Check sheet for the drawn part. Datum: minimum x, y, z corner. Units: mm. A direction names the side the tool comes from. Give positions to 0.01 mm unless a question says otherwise; leave off trailing zeros. Order: outer loops, then holes, each group sorted by start corner. A loop starts at its lowest first (then second) coordinate and runs counter-clockwise, first axis right, second up.
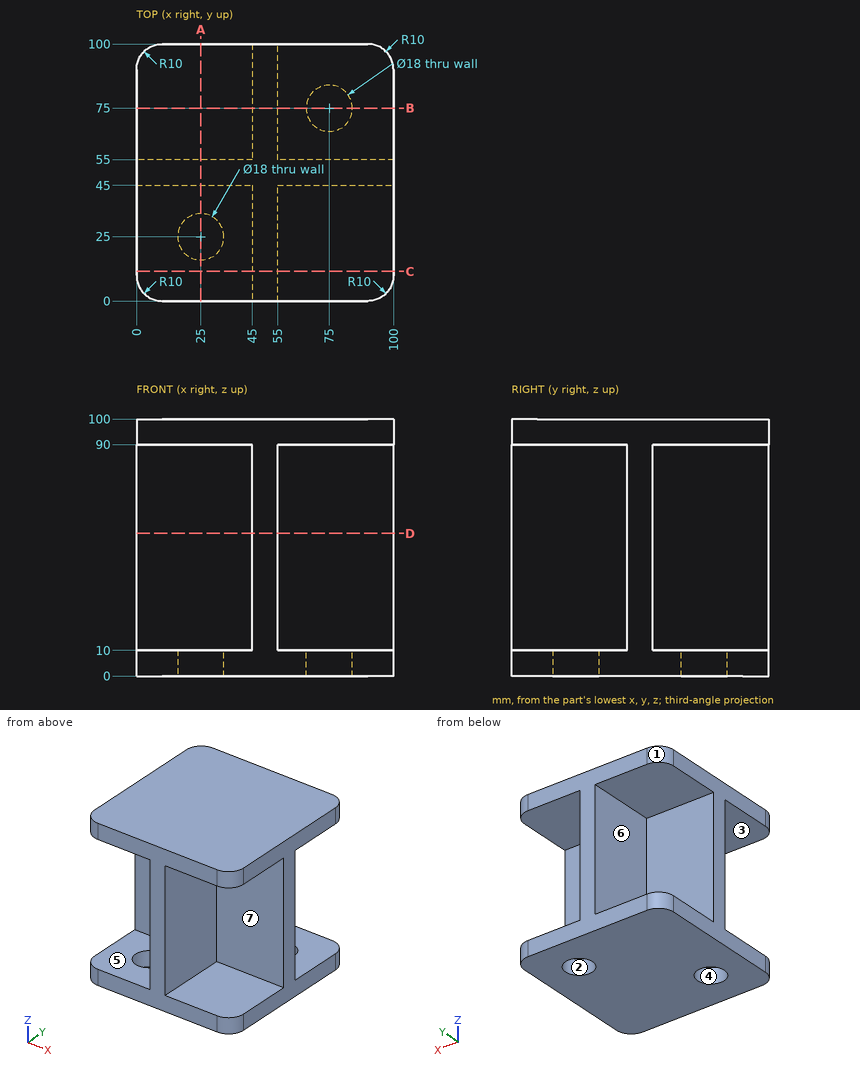
Q1. Sectioned sample at C-C, the plane y = 11.5. Record the cut outline in (x, z), plus the area to 3 significant figures.
Q2. Draft check along X on the marked faces 1, 2 and 3. Enter one of: pulls with the +X half, pulls with the -X half, needs draft (parallel to the pull), parting line crosses it, or undercut.
Q3. Go/stop test with a flat-tipped pin: P1, Ø8, axis at y = 81, z = 84, coming from the -X side. Record where the tip stops, or that it passes through.
Q4. Sectioned sample at B-B, the plane y = 75. Record the cut outline in (x, z), plus the area to 3 significant figures.
Q5. Sectioned sample at D-D, the plane z = 55.5. Record the cut outline in (x, y).
Q6. Sectioned sample at A-A, the plane x = 25. Record the cut outline in (y, z), plus the area to 3 significant figures.
Q7. Material ranges on line 1 (Z direction, x = 79, y = 89); line 2 (X direction, y = 25, z = 7); line 3 (Y direction, x = 75, z = 6.75), recorded low to high.
Q8. Tool access check on the marked faces 4, 5, 6 and 7. Record the directions out of +Z, -Z, +X, -X, +Y, -Y that give a thin tool (end or side, any length) a straight path to the whole face; none if there is none.
Filled in:
1. outline: (0, 0) - (100, 0) - (100, 10) - (55, 10) - (55, 90) - (100, 90) - (100, 100) - (0, 100) - (0, 90) - (45, 90) - (45, 10) - (0, 10) - close
1. area: 2,800 mm2
2. face 1: pulls with the -X half
2. face 2: undercut
2. face 3: needs draft
3. P1: stops at x = 45
4. outline: (0, 0) - (66, 0) - (66, 10) - (55, 10) - (55, 90) - (100, 90) - (100, 100) - (0, 100) - (0, 90) - (45, 90) - (45, 10) - (0, 10) - close; (84, 0) - (100, 0) - (100, 10) - (84, 10) - close
4. area: 2,620 mm2
5. outline: (0, 45) - (45, 45) - (45, 0) - (55, 0) - (55, 45) - (100, 45) - (100, 55) - (55, 55) - (55, 100) - (45, 100) - (45, 55) - (0, 55) - close
6. outline: (0, 0) - (16, 0) - (16, 10) - (0, 10) - close; (0, 90) - (45, 90) - (45, 10) - (34, 10) - (34, 0) - (100, 0) - (100, 10) - (55, 10) - (55, 90) - (100, 90) - (100, 100) - (0, 100) - close
6. area: 2,620 mm2
7. line 1: z = 0 to 10, 90 to 100
7. line 2: x = 0 to 16, 34 to 100
7. line 3: y = 0 to 66, 84 to 100
8. face 4: -Z
8. face 5: -X, -Y
8. face 6: -X, +Y
8. face 7: +X, -Y
